```python
from build123d import *

# Parameters (mm, degrees)
SKETCH2_W               = 533.4
SKETCH2_H               = 609.6
SKETCH2_W_2             = 101.6
SKETCH2_H_2             = 25.4
BOSS_EXTRUDE1_DEPTH     = 17.78
SKETCH3_W               = 101.6
SKETCH3_H               = 25.4
BOSS_EXTRUDE2_DEPTH     = 17.78
SKETCH3_2_W             = 101.6
SKETCH3_2_H             = 25.4
BOSS_EXTRUDE3_DEPTH     = 292.1
CUT_EXTRUDE1_DEPTH      = 508
CUT_EXTRUDE1_DEPTH_BACK = 508
SKETCH4_R               = 12.7
SKETCH5_W               = 17.78
SKETCH5_H               = 609.6
BOSS_EXTRUDE4_DEPTH     = 381


with BuildPart() as part:
    # Sketch2 → Boss-Extrude1 (new body)
    with BuildSketch(Plane(origin=(0, 0, 0), x_dir=(1, 0, 0), z_dir=(0, 1, 0))):
        Rectangle(SKETCH2_W, SKETCH2_H)
        with Locations((0, -266.7)):
            Rectangle(SKETCH2_W_2, SKETCH2_H_2, mode=Mode.SUBTRACT)
        with Locations((0, 266.7)):
            Rectangle(SKETCH2_W_2, SKETCH2_H_2, mode=Mode.SUBTRACT)
    extrude(amount=BOSS_EXTRUDE1_DEPTH)

    # Sketch3 → Boss-Extrude2 (add)
    with BuildSketch(Plane(origin=(0, 0, 0), x_dir=(1, 0, 0), z_dir=(0, 1, 0))):
        with Locations((0, -266.7)):
            Rectangle(SKETCH3_W, SKETCH3_H)
        with Locations((0, 266.7)):
            Rectangle(SKETCH3_W, SKETCH3_H)
    extrude(amount=BOSS_EXTRUDE2_DEPTH)

    # Sketch3_2 → Boss-Extrude3 (add)
    with BuildSketch(Plane(origin=(0, 0, 0), x_dir=(1, 0, 0), z_dir=(0, 1, 0))):
        with Locations((0, -266.7)):
            Rectangle(SKETCH3_2_W, SKETCH3_2_H)
        with Locations((0, 266.7)):
            Rectangle(SKETCH3_2_W, SKETCH3_2_H)
    extrude(amount=-BOSS_EXTRUDE3_DEPTH)

    # Sketch4 → Cut-Extrude1 (cut, two sides: drawn at the far end of the back side and taken through both)
    with BuildSketch(Plane.XY.offset(-CUT_EXTRUDE1_DEPTH_BACK)):
        with Locations(Location((0, -266.7, 0), (0, 0, 180))):
            Circle(SKETCH4_R)
    extrude(amount=CUT_EXTRUDE1_DEPTH + CUT_EXTRUDE1_DEPTH_BACK, mode=Mode.SUBTRACT)

    # Sketch5 → Boss-Extrude4 (add)
    with BuildSketch(Plane(origin=(0, 0, 0), x_dir=(1, 0, 0), z_dir=(0, 1, 0))):
        with Locations((-257.81, 0)):
            Rectangle(SKETCH5_W, SKETCH5_H)
    extrude(amount=-BOSS_EXTRUDE4_DEPTH)


solid = part.part
```
Design review of the part built by this model. Coordinates are the model's own, in mm. A direction names the side the tool comes from. Coordinates: 2 decimals unless noted, no trailing zeros. Write each loop counter-clockwise with the first axis right and the second up, starting at its lowest first coordinate (ties: lowest second). Pieces come first, ordered by that corner, then holes.
1) To check wall thickness, follow L1, parallel to X at y = -266, z = 259; L2, parallel to Y at x = 0, z = 262; L3, parallel to Z at x = 20, y = -112.5. State the ranges of each line that lie inside material, in increasing order.
2) Add section A-A (y = -133.5). Write out the cut boundary in (x, z), plus the area to 3 significant figures.
3) Mouldability with a two-part tool opening along X and no side actions: class faces 5 (the flat face through (-4, 17.78, -4)), 6 (the flat face through (-266.7, -179, 4)), 7 (the flat face through (50.8, -144, 267)), 8 (the cylindrical face through (2.75, -254.3, -266.88)) as +X half, -X half, draft (parallel to the pull), parting line (faces both ways), or undercut.
4) Add section B-B (x = 0). Write out the cut boundary in (y, z), plus the area to 3 significant figures.
5) Machinability: for faces 1 (the flat face through (-1, -292.1, 267)), 2 (the flat face through (-248.92, -188, 4)), 3 (the flat face through (-1, -144, -254)), 4 (the flat face through (-1, -144, 279.4)), which of the approach directions +Z, -Z, +X, -X, +Y, -Y give a long, thin tool a straight path to every point of the face, cutting with its end or side? Answer none if there is none.
6) Add section D-D (z = 49). Write out the cut boundary in (x, y), plus the area to 3 significant figures.
7) Add section C-C (y = -266.7). Write out the cut boundary in (x, z).
8) Insertion check: pin 1 (6 mm diameter, centred on y = -313.5, z = -115, fed in from +X); pin 2 (7.5 mm diameter, centred on y = -131.5, z = -272.5, fed in from +X); pin 3 (20.5 mm diameter, centred on x = 4.5, z = -272, fed in from -Y). Each pin has a flat end and moves straight along its axis. Give the tip position at first contact, or say it passes through.
Check result:
1. L1: x = -266.7 to -248.92, -50.8 to -12.68, 12.68 to 50.8
1. L2: y = -292.1 to -279.4, -254 to 17.78
1. L3: z = -279.4 to -254, 254 to 279.4
2. outline: (-266.7, -304.8) - (-248.92, -304.8) - (-248.92, 304.8) - (-266.7, 304.8) - close; (-50.8, -279.4) - (50.8, -279.4) - (50.8, -254) - (-50.8, -254) - close; (-50.8, 254) - (50.8, 254) - (50.8, 279.4) - (-50.8, 279.4) - close
2. area: 16,000 mm2
3. face 5: draft
3. face 6: -X half
3. face 7: +X half
3. face 8: undercut
4. outline: (-292.1, -279.4) - (-279.4, -279.4) - (-279.4, -254) - (-292.1, -254) - close; (-292.1, 254) - (-279.4, 254) - (-279.4, 279.4) - (-292.1, 279.4) - close; (-254, -279.4) - (0, -279.4) - (0, -304.8) - (17.78, -304.8) - (17.78, 304.8) - (0, 304.8) - (0, 279.4) - (-254, 279.4) - (-254, 254) - (0, 254) - (0, -254) - (-254, -254) - close
4. area: 24,400 mm2
5. face 1: +Z, -Z, +X, -Y
5. face 2: +Z, -Z, -Y
5. face 3: +X, -Y
5. face 4: +Z, +X, -Y
6. outline: (-266.7, -381) - (-248.92, -381) - (-248.92, 0) - (266.7, 0) - (266.7, 17.78) - (-266.7, 17.78) - close
6. area: 16,300 mm2
7. outline: (-266.7, -304.8) - (-248.92, -304.8) - (-248.92, 304.8) - (-266.7, 304.8) - close; (-50.8, -279.4) - (-12.7, -279.4) - (-12.7, -254) - (-50.8, -254) - close; (-50.8, 254) - (-12.7, 254) - (-12.7, 279.4) - (-50.8, 279.4) - close; (12.7, -279.4) - (50.8, -279.4) - (50.8, -254) - (12.7, -254) - close; (12.7, 254) - (50.8, 254) - (50.8, 279.4) - (12.7, 279.4) - close
8. pin 1: stops at x = -248.92
8. pin 2: stops at x = 50.8
8. pin 3: stops at y = -292.1
